Read the model definition and answer for the solid it produces. Units are mm, in the model's axes. Face numbers are marked on the shaded views. A direction names the side the tool comes from. Round coordinates to 2 decimals unless told otherwise and drop trailing zeros. Write each loop counter-clockwise with the first axis right and the second up, starting at its lowest first coordinate (ties: lowest second). Pieces come first, ordered by that corner, then holes.
from build123d import *

# Parameters (mm, degrees)
SALIENTE_EXTRUIR2_DEPTH = 3
CROQUIS3_R              = 3.25
CROQUIS3_R_2            = 1.65
CORTAR_EXTRUIR1_DEPTH   = 3
REDONDEO1_R             = 1.5
REDONDEO2_R             = 1.5
REDONDEO3_R             = 1.5
REDONDEO4_R             = 1.5


with BuildPart() as part:
    # Croquis1 → Saliente-Extruir2 (new body)
    with BuildSketch(Plane.XY):
        with BuildLine():
            Line((-7.7, 3.7), (-24.7, 3.7))
            ThreePointArc((-24.7, 3.7), (-28.4, 0), (-24.7, -3.7))
            Line((-24.7, -3.7), (-7.7, -3.7))
            ThreePointArc((-7.7, -3.7), (-4.871572875, -4.871572875), (-3.7, -7.7))
            Line((-3.7, -7.7), (-3.7, -24.7))
            ThreePointArc((-3.7, -24.7), (0, -28.4), (3.7, -24.7))
            Line((3.7, -24.7), (3.7, -7.7))
            ThreePointArc((3.7, -7.7), (4.871572875, -4.871572875), (7.7, -3.7))
            Line((7.7, -3.7), (24.7, -3.7))
            ThreePointArc((24.7, -3.7), (28.4, 0), (24.7, 3.7))
            Line((24.7, 3.7), (7.7, 3.7))
            ThreePointArc((7.7, 3.7), (4.871572875, 4.871572875), (3.7, 7.7))
            Line((3.7, 7.7), (3.7, 24.7))
            ThreePointArc((3.7, 24.7), (0, 28.4), (-3.7, 24.7))
            Line((-3.7, 24.7), (-3.7, 7.7))
            ThreePointArc((-3.7, 7.7), (-4.871572875, 4.871572875), (-7.7, 3.7))
        make_face()
    extrude(amount=SALIENTE_EXTRUIR2_DEPTH)

    # Croquis3 → Cortar-Extruir1 (cut)
    with BuildSketch(Plane.XY.offset(3)):
        Circle(CROQUIS3_R)
        with Locations((-7.5, 0)):
            Circle(CROQUIS3_R_2)
        with Locations((-22.5, 0)):
            Circle(CROQUIS3_R_2)
        with Locations((0, -9.5)):
            Circle(CROQUIS3_R_2)
        with Locations((7.5, 0)):
            Circle(CROQUIS3_R_2)
        with Locations((0, 9.5)):
            Circle(CROQUIS3_R_2)
        with Locations((0, 24.5)):
            Circle(CROQUIS3_R_2)
        with Locations((22.5, 0)):
            Circle(CROQUIS3_R_2)
        with Locations((0, -24.5)):
            Circle(CROQUIS3_R_2)
    extrude(amount=-CORTAR_EXTRUIR1_DEPTH, mode=Mode.SUBTRACT)

    # Redondeo1
    redondeo1_edges = [part.edges().sort_by_distance(p)[0] for p in [
        (-9.15, 0, 3),
    ]]
    fillet(redondeo1_edges, radius=REDONDEO1_R)

    # Redondeo2
    redondeo2_edges = [part.edges().sort_by_distance(p)[0] for p in [
        (-1.65, 9.5, 3),
    ]]
    fillet(redondeo2_edges, radius=REDONDEO2_R)

    # Redondeo3
    redondeo3_edges = [part.edges().sort_by_distance(p)[0] for p in [
        (5.85, 0, 3),
    ]]
    fillet(redondeo3_edges, radius=REDONDEO3_R)

    # Redondeo4
    redondeo4_edges = [part.edges().sort_by_distance(p)[0] for p in [
        (-1.65, -9.5, 3),
    ]]
    fillet(redondeo4_edges, radius=REDONDEO4_R)


solid = part.part
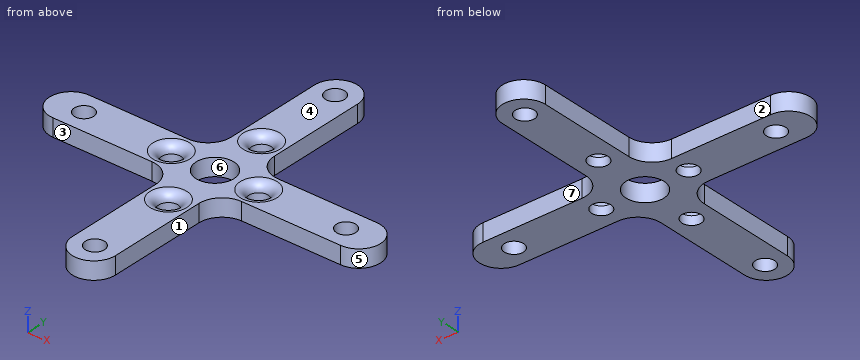
Q1. Section C-C (y = -9.5) is taken. Determine the outline of the cut face in (x, z), then the cut area to 3 significant figures.
Verdict:
outline: (-3.7, 0) - (-1.65, 0) - (-1.65, 1.5) arc R1.5 ccw to (-3.15, 3) - (-3.7, 3) - close; (1.65, 0) - (3.7, 0) - (3.7, 3) - (3.15, 3) arc R1.5 ccw to (1.65, 1.5) - close
area: 11.3 mm2
Q2. Section A-A (x = -22.5) is taken. Determine the outline of the cut face in (y, z), then the cut area to 3 significant figures.
Verdict:
outline: (-3.7, 0) - (-1.65, 0) - (-1.65, 3) - (-3.7, 3) - close; (1.65, 0) - (3.7, 0) - (3.7, 3) - (1.65, 3) - close
area: 12.3 mm2
Q3. Which of the six approach directions +Z, -Z, +X, -X, +Y, -Y give full straight-line access (tool end or side, diameter ignored) to the marked faces 1, 2 and 3?
Verdict:
face 1: +Z, -Z, +X, -Y
face 2: +Z, -Z, -X, +Y
face 3: +Z, -Z, -X, -Y
Q4. Section D-D (x = 0) is taken. Determine the outline of the cut face in (y, z), then the cut area to 3 significant figures.
Verdict:
outline: (-28.4, 0) - (-26.15, 0) - (-26.15, 3) - (-28.4, 3) - close; (-22.85, 0) - (-11.15, 0) - (-11.15, 1.5) arc R1.5 ccw to (-12.65, 3) - (-22.85, 3) - close; (-7.85, 0) - (-3.25, 0) - (-3.25, 3) - (-6.35, 3) arc R1.5 ccw to (-7.85, 1.5) - close; (3.25, 0) - (7.85, 0) - (7.85, 1.5) arc R1.5 ccw to (6.35, 3) - (3.25, 3) - close; (11.15, 0) - (22.85, 0) - (22.85, 3) - (12.65, 3) arc R1.5 ccw to (11.15, 1.5) - close; (26.15, 0) - (28.4, 0) - (28.4, 3) - (26.15, 3) - close
area: 109 mm2
Q5. Straight lines are drawn through the part: probe 1 along Y at (x, z) = (0, 1.85); probe 2 along X at (y, z) = (-20, 2.85); probe 3 along Y at (x, z) = (22.5, 1.95). For each, find the intervals that lie inside material, in ascending order.
Verdict:
probe 1: y = -28.4 to -26.15, -22.85 to -11.19, -7.81 to -3.25, 3.25 to 7.81, 11.19 to 22.85, 26.15 to 28.4
probe 2: x = -3.7 to 3.7
probe 3: y = -3.7 to -1.65, 1.65 to 3.7
Q6. Flat-ended cylindrical pins translate along their axes: pin 1 Ø4 at (x, y) = (0, 0) entering from +Z; pin 2 Ø4.5 at (x, y) = (0, 9.5) entering from +Z; pin 3 Ø4 at (x, y) = (7.5, 0) entering from +Z; pin 4 Ø0.9 at (x, z) = (-12, 2) entering from -Y. Find the tip coordinate at first contact, or state that the pin passes through.
Verdict:
pin 1: passes through
pin 2: stops at z = 2.7
pin 3: stops at z = 2.46
pin 4: stops at y = -3.7
Q7. Section B-B (z = 0.8) is taken. State how many separate pieces and enclosed holes the cut face has, then the cut area to 3 significant figures.
Verdict:
separate pieces: 1
enclosed holes: 9
area: 675 mm2
Q8. Determine the mould class of the marked faces 4, 5, 6 and 7 for opening direction Y: pulls with the +Y half, pulls with the -Y half, needs draft (parallel to the pull), parting line crosses it, or undercut.
Verdict:
face 4: needs draft
face 5: parting line crosses it
face 6: undercut
face 7: pulls with the +Y half
